Check sheet for the modelled part. Datum: model origin and axes. Units: mm. Round coordinates to 2 decimals unless told otherwise and drop trailing zeros. Order: outer loops, then holes, each group sorted by start corner. A loop starts at its lowest first (then second) coordinate and runs counter-clockwise, first axis right, second up. Notation, with made-up numbers: (42, 78) -> (63, 78) arc R15 ccw to (63, 88) -> close; hole circle Ø1 at (-30.75, 38). An arc over 180 degrees is marked (long way). Answer in a Markdown table with one row per item.
```python
from build123d import *

# Parameters (mm, degrees)
SKETCH1_R                     = 3.5
BOSS_EXTRUDE1_DEPTH           = 27
BOSS_EXTRUDE1_TAPER           = 1.15
BOSS_EXTRUDE1_OTHER_WAY_DEPTH = 27
BOSS_EXTRUDE1_OTHER_WAY_TAPER = -1.15


with BuildPart() as part:
    # Sketch1 → Boss-Extrude1 (new body)
    with BuildSketch(Plane(origin=(0, 0, 0), x_dir=(0, 0, -1), z_dir=(1, 0, 0))):
        Circle(SKETCH1_R)
    extrude(amount=BOSS_EXTRUDE1_DEPTH, taper=BOSS_EXTRUDE1_TAPER)

    # Sketch1 → Boss-Extrude1 other way (add)
    with BuildSketch(Plane(origin=(0, 0, 0), x_dir=(0, 0, -1), z_dir=(1, 0, 0))):
        Circle(SKETCH1_R)
    extrude(amount=-BOSS_EXTRUDE1_OTHER_WAY_DEPTH, taper=BOSS_EXTRUDE1_OTHER_WAY_TAPER)

    # Fillet1
    # an asymmetric fillet: 3.7, 1 mm, written as the material it takes off along each edge
    with BuildSketch(Plane(origin=(-27, 0, 0), x_dir=(0, 0, -1), z_dir=(0, -1, 0))) as fillet1_piece_1:
        with BuildLine():
            Bezier((4.020432866, 1.074258773), (4.041997517, 0), (0.321178125, 0), weights=[1, 0.699975021, 1])
            Line((0.321178125, 0), (4.041997517, 0))
            Line((4.041997517, 0), (4.020432866, 1.074258773))
        make_face()
    revolve(axis=Axis((-27, 0, 0), (1, 0, 0)), mode=Mode.SUBTRACT)

    # Fillet2
    # an asymmetric fillet: 2.8, 1 mm, written as the material it takes off along each edge
    with BuildSketch(Plane(origin=(27, 0, 0), x_dir=(0, 0, -1), z_dir=(0, 1, 0))) as fillet2_piece_1:
        with BuildLine():
            Bezier((2.976948391, 0.943804171), (2.958002483, 0), (0.177512371, 0), weights=[1, 0.714167326, 1])
            Line((0.177512371, 0), (2.958002483, 0))
            Line((2.958002483, 0), (2.976948391, 0.943804171))
        make_face()
    revolve(axis=Axis((27, 0, 0), (-1, 0, 0)), mode=Mode.SUBTRACT)


solid = part.part
```
(1) Section check A-A on x = 18. Record the boundary of the cut face in (y, z).
Solutions:
| item | result |
|---|---|
| outline | circle Ø6.28 at (0, 0) |
(2) Depth check by flat-ended pin: pin 1 Ø1 at (x, z) = (17, -2.5) entering from -Y; pin 2 Ø1 at (x, y) = (11.5, 2) entering from -Z; pin 3 Ø1 at (y, z) = (2, 1.5) entering from -X. Enter the tip coordinate at first touch or a pass-through.
Solutions:
| item | result |
|---|---|
| pin 1 | y = -2.45 |
| pin 2 | z = -2.9 |
| pin 3 | x = -26.88 |
(3) Section check B-B on x = -17. Record the boundary of the cut face in (y, z), plus the area to 3 significant figures.
Solutions:
| item | result |
|---|---|
| outline | circle Ø7.68 at (0, 0) |
| area | 46.4 mm^2 |
(4) Scan lines: probe 1 along Y at (x, z) = (-11, 1.5); probe 2 along Z at (x, y) = (20, -1); probe 3 along Y at (x, z) = (12, -3). Record each from-to range of solid material in increasing order. Write a range as from..to.
Solutions:
| item | result |
|---|---|
| probe 1 | -3.41..3.41 |
| probe 2 | -2.93..2.93 |
| probe 3 | -1.27..1.27 |
